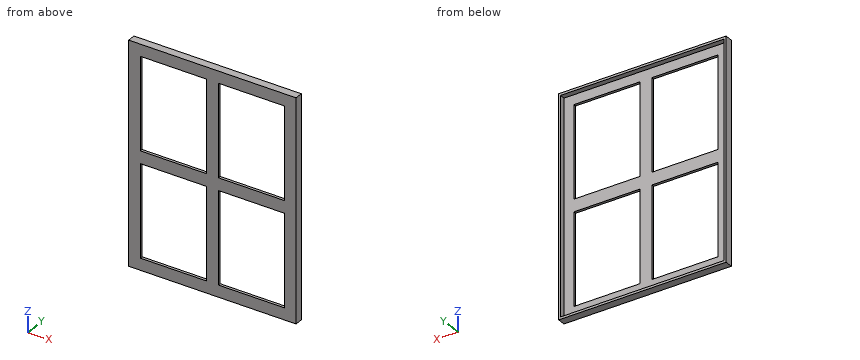
```python
from build123d import *

# Parameters (mm, degrees)
CROQUIS1_W              = 620
CROQUIS1_H              = 820
SALIENTE_EXTRUIR1_DEPTH = 10
CROQUIS2_W              = 633.624968344
CROQUIS2_H              = 837.075812624
CROQUIS2_W_2            = 620
CROQUIS2_H_2            = 820
SALIENTE_EXTRUIR2_DEPTH = 20
CROQUIS3_W              = 633.624968344
CROQUIS3_H              = 837.075812624
SALIENTE_EXTRUIR3_DEPTH = 10
CROQUIS4_W              = 250
CROQUIS4_H              = 350
CORTAR_EXTRUIR1_DEPTH   = 10


with BuildPart() as part:
    # Croquis1 → Saliente-Extruir1 (new body)
    with BuildSketch(Plane(origin=(0, 0, 0), x_dir=(1, 0, 0), z_dir=(0, 1, 0))):
        Rectangle(CROQUIS1_W, CROQUIS1_H)
    extrude(amount=SALIENTE_EXTRUIR1_DEPTH)



with BuildPart() as body_2:
    # Croquis2 → Saliente-Extruir2 (new body)
    with BuildSketch(Plane(origin=(0, 10, 0), x_dir=(1, 0, 0), z_dir=(0, 1, 0))):
        Rectangle(CROQUIS2_W, CROQUIS2_H)
        Rectangle(CROQUIS2_W_2, CROQUIS2_H_2, mode=Mode.SUBTRACT)
    extrude(amount=SALIENTE_EXTRUIR2_DEPTH)


with BuildPart() as part_1:
    add(part.part)

    add(body_2.part)  # Saliente-Extruir3 merges body 2
    # Croquis3 → Saliente-Extruir3 (add)
    with BuildSketch(Plane.XZ.offset(-10)):
        Rectangle(CROQUIS3_W, CROQUIS3_H)
    extrude(amount=SALIENTE_EXTRUIR3_DEPTH)

    # Croquis4 → Cortar-Extruir1 (cut)
    with BuildSketch(Plane.XZ):
        with Locations((-147.812484172, 198.537906312)):
            Rectangle(CROQUIS4_W, CROQUIS4_H)
        with Locations((147.812484172, 198.537906312)):
            Rectangle(CROQUIS4_W, CROQUIS4_H)
        with Locations((-147.812484172, -198.537906312)):
            Rectangle(CROQUIS4_W, CROQUIS4_H)
        with Locations((147.812484172, -198.537906312)):
            Rectangle(CROQUIS4_W, CROQUIS4_H)
    extrude(amount=-CORTAR_EXTRUIR1_DEPTH, mode=Mode.SUBTRACT)


solid = part_1.part
```
For this review, take the finished solid that the model builds, in its own axes (mm). Round coordinates to 2 decimals unless told otherwise and drop trailing zeros. Loops run counter-clockwise (first coordinate to the right, second up) from the corner with the lowest first, then second, coordinate; pieces in that order, holes last.
Q1. To check wall thickness, follow line 1 along Z through (x, y) = (101, 5); line 2 along X through (y, z) = (3.5, -82); line 3 along X through (y, z) = (10.75, -292.5). State the ranges of each line that lie inside material, in increasing order.
Result sheet:
line 1: z = -418.54 to -373.54, -23.54 to 23.54, 373.54 to 418.54
line 2: x = -316.81 to -272.81, -22.81 to 22.81, 272.81 to 316.81
line 3: x = -316.81 to -310, 310 to 316.81
Q2. Add section B-B on x = -98.5. Write out the cut boundary in (y, z).
Result sheet:
outline: (0, -418.54) - (30, -418.54) - (30, -410) - (10, -410) - (10, -373.54) - (0, -373.54) - close; (0, -23.54) - (10, -23.54) - (10, 23.54) - (0, 23.54) - close; (0, 373.54) - (10, 373.54) - (10, 410) - (30, 410) - (30, 418.54) - (0, 418.54) - close
Q3. Add section A-A on z = -339.5. Write out the cut boundary in (x, y), plus the area to 3 significant figures.
Result sheet:
outline: (-316.81, 0) - (-272.81, 0) - (-272.81, 10) - (-310, 10) - (-310, 30) - (-316.81, 30) - close; (-22.81, 0) - (22.81, 0) - (22.81, 10) - (-22.81, 10) - close; (272.81, 0) - (316.81, 0) - (316.81, 30) - (310, 30) - (310, 10) - (272.81, 10) - close
area: 1,610 mm2
Q4. Insertion check: pin 1 Ø1 at (x, z) = (102, 15) entering from +Y. The pin has a flat end and moves straight along its axis. Give the tip position at first contact, or say it passes through.
Result sheet:
pin 1: stops at y = 10
Q5. Add section C-C on y = 20.25. Write out the cut boundary in (x, z).
Result sheet:
outline: (-316.81, -418.54) - (316.81, -418.54) - (316.81, 418.54) - (-316.81, 418.54) - close; hole (-310, -410) - (310, -410) - (310, 410) - (-310, 410) - close
